Source: three-view drawing plus pictorial views. Frame: mm from the lowest corner of the part. A direction names the side the tool comes from. Round coordinates to 2 decimals unless told otherwise and drop trailing zeros. Order: outer loops, then holes, each group sorted by start corner. A loop starts at its lowest first (then second) coordinate and runs counter-clockwise, first axis right, second up. Notation, with made-up numbers: (44, 2.5) -> (63, 2.5) arc R19 ccw to (63, 31.5) -> close; hole circle Ø10 at (12, -15). An arc over 180 degrees is marked (long way). Use a Markdown table: item, result.
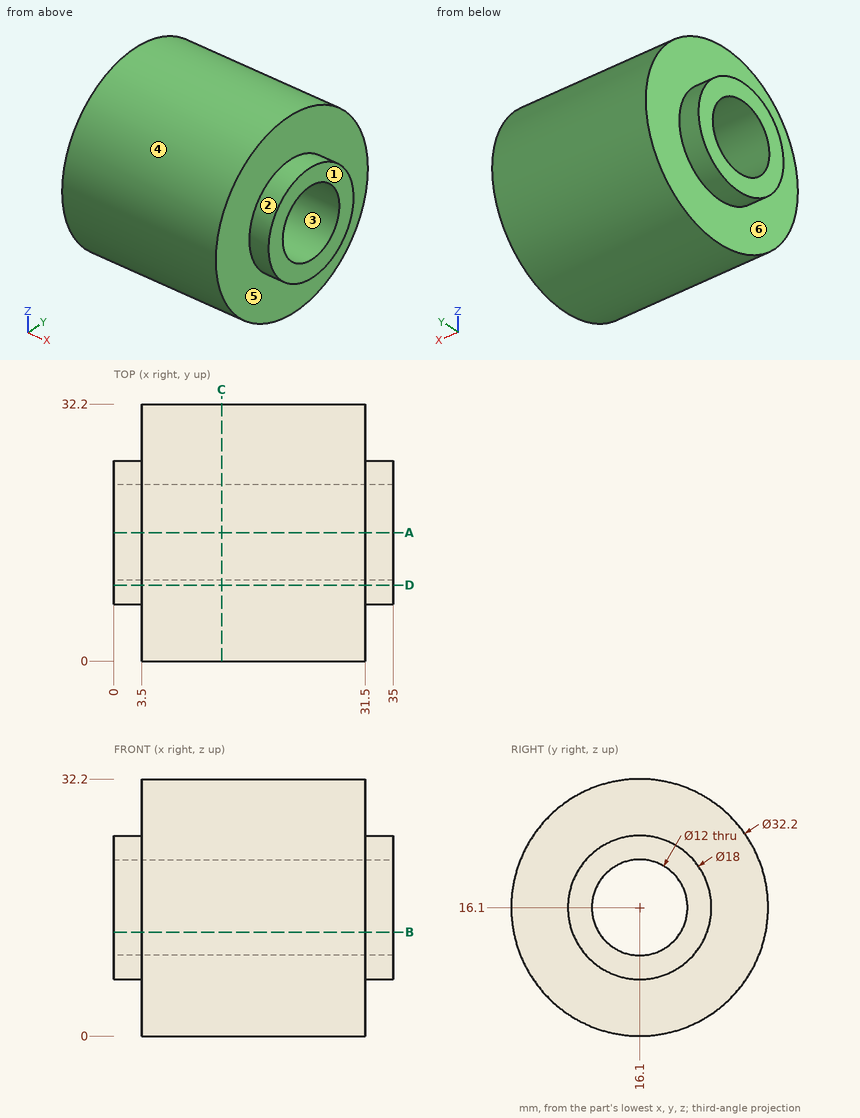
1) Cut plane D-D on y = 9.5. Return loops of the section in (x, z), and give its area (3 significant figures).
Results found:
| item | result |
|---|---|
| outline | (0, 9.98) -> (3.5, 9.98) -> (3.5, 1.41) -> (31.5, 1.41) -> (31.5, 9.98) -> (35, 9.98) -> (35, 22.22) -> (31.5, 22.22) -> (31.5, 30.79) -> (3.5, 30.79) -> (3.5, 22.22) -> (0, 22.22) -> close |
| area | 908 mm² |
2) Cut plane B-B on z = 13. Return loops of the section in (x, y).
Results found:
| item | result |
|---|---|
| outline | (0, 7.65) -> (3.5, 7.65) -> (3.5, 0.3) -> (31.5, 0.3) -> (31.5, 7.65) -> (35, 7.65) -> (35, 10.96) -> (0, 10.96) -> close; (0, 21.24) -> (35, 21.24) -> (35, 24.55) -> (31.5, 24.55) -> (31.5, 31.9) -> (3.5, 31.9) -> (3.5, 24.55) -> (0, 24.55) -> close |
3) Pin query (flat end, axial travel): pin 1 Ø1.5 at (x, z) = (18, 23.5) entering from -Y; pin 2 Ø5 at (x, z) = (20.5, 6) entering from +Y; pin 3 Ø8 at (y, z) = (7, 28) entering from +X; pin 4 Ø10 at (x, z) = (13, 11) entering from +Y. Return the tip coordinate at first contact, or that it passes through.
Results found:
| item | result |
|---|---|
| pin 1 | stops at y = 1.44 |
| pin 2 | stops at y = 30.29 |
| pin 3 | stops at x = 31.5 |
| pin 4 | stops at y = 32.2 |
4) Set-up query: the marked faces 4, 5 and 6. Return all of +Z, -Z, +X, -X, +Y, -Y with unobstructed straight access to the full face (end or side cutting, diameter ignored); none if empty.
Results found:
| item | result |
|---|---|
| face 4 | +X, -X |
| face 5 | +X |
| face 6 | -X |
5) Line query: L1, parallel to Y at x = 19.5, z = 16.1; L2, parallel to X at y = 22.5, z = 27. Output: solid intervals per line, ascending. Write a range as [from, to].
Results found:
| item | result |
|---|---|
| L1 | y = [0, 10.1], [22.1, 32.2] |
| L2 | x = [3.5, 31.5] |
6) Cut plane A-A on y = 16.1. Return loops of the section in (x, z), and give its area (3 significant figures).
Results found:
| item | result |
|---|---|
| outline | (0, 7.1) -> (3.5, 7.1) -> (3.5, 0) -> (31.5, 0) -> (31.5, 7.1) -> (35, 7.1) -> (35, 10.1) -> (0, 10.1) -> close; (0, 22.1) -> (35, 22.1) -> (35, 25.1) -> (31.5, 25.1) -> (31.5, 32.2) -> (3.5, 32.2) -> (3.5, 25.1) -> (0, 25.1) -> close |
| area | 608 mm² |
7) Cut plane C-C on x = 13.5. Return loops of the section in (y, z).
Results found:
| item | result |
|---|---|
| outline | circle Ø32.2 at (16.1, 16.1); hole circle Ø12 at (16.1, 16.1) |
8) Pull-direction query (Z, two-part tool) for the marked faces 1, 2 and 3; classes: +Z half, -Z half, draft (parallel to the pull), parting line (faces both ways), or undercut.
Results found:
| item | result |
|---|---|
| face 1 | draft |
| face 2 | parting line |
| face 3 | undercut |
